```python
from build123d import *

# Parameters (mm, degrees)
SKETCH1_R           = 12.1
BOSS_EXTRUDE1_DEPTH = 31
SKETCH2_R           = 12.65
BOSS_EXTRUDE2_DEPTH = 19
SKETCH3_R           = 3.5
BOSS_EXTRUDE3_DEPTH = 2
SKETCH4_R           = 2
BOSS_EXTRUDE4_DEPTH = 12
SKETCH5_R           = 1.5
CUT_EXTRUDE1_DEPTH  = 6
CUT_EXTRUDE2_START  = -10
CUT_EXTRUDE2_DEPTH  = 10


with BuildPart() as part:
    # Sketch1 → Boss-Extrude1 (new body)
    with BuildSketch(Plane(origin=(0, 0, 0), x_dir=(1, 0, 0), z_dir=(0, 1, 0))):
        with Locations(Location((0, 0, 0), (0, 0, 270))):
            Circle(SKETCH1_R)
    extrude(amount=BOSS_EXTRUDE1_DEPTH)

    # Sketch2 → Boss-Extrude2 (add)
    with BuildSketch(Plane(origin=(0, 31, 0), x_dir=(1, 0, 0), z_dir=(0, 1, 0))):
        with Locations(Location((0, 0, 0), (0, 0, 270))):
            Circle(SKETCH2_R)
    extrude(amount=BOSS_EXTRUDE2_DEPTH)

    # Sketch3 → Boss-Extrude3 (add)
    with BuildSketch(Plane(origin=(0, 50, 0), x_dir=(1, 0, 0), z_dir=(0, 1, 0))):
        with Locations(Location((0, 0, 0), (0, 0, 270))):
            Circle(SKETCH3_R)
    extrude(amount=BOSS_EXTRUDE3_DEPTH)

    # Sketch4 → Boss-Extrude4 (add)
    with BuildSketch(Plane(origin=(0, 52, 0), x_dir=(1, 0, 0), z_dir=(0, 1, 0))):
        with Locations(Location((0, 0, 0), (0, 0, 270))):
            Circle(SKETCH4_R)
    extrude(amount=BOSS_EXTRUDE4_DEPTH)

    # Sketch5 → Cut-Extrude1 (cut)
    with BuildSketch(Plane(origin=(0, 50, 0), x_dir=(1, 0, 0), z_dir=(0, 1, 0))):
        with Locations(Location((8.25, 0, 0), (0, 0, 270))):
            Circle(SKETCH5_R)
        with Locations(Location((-8.25, 0, 0), (0, 0, 270))):
            Circle(SKETCH5_R)
    extrude(amount=-CUT_EXTRUDE1_DEPTH, mode=Mode.SUBTRACT)

    # Sketch6 → Cut-Extrude2 (cut)
    with BuildSketch(Plane(origin=(0, 64, 0), x_dir=(1, 0, 0), z_dir=(0, 1, 0)).offset(CUT_EXTRUDE2_START)):
        with BuildLine():
            Line((-1.428285686, 1.4), (1.428285686, 1.4))
            ThreePointArc((1.428285686, 1.4), (0, 2), (-1.428285686, 1.4))
        make_face()
    extrude(amount=CUT_EXTRUDE2_DEPTH, mode=Mode.SUBTRACT)


solid = part.part
```
Input: part model. Units: mm. Frame: model coordinates. A direction names the side the tool comes from. Give positions to 0.01 mm unless a question says otherwise; leave off trailing zeros. Loops run counter-clockwise (first coordinate to the right, second up) from the corner with the lowest first, then second, coordinate; pieces in that order, holes last. Notation, with made-up numbers: M 16.5,22 L 70.5,22 A25 cw 70.5,44 Z; hole C 4.5,71 d11. An arc over 180 degrees is marked long. Answer as CSV lines item,"result". Start each with the question number.
1. Section B-B on z = -9. Return loops of the section in (x, y).
2. Pull-direction query (X, two-part tool) for faces 5 (the face through (-0.766, 57.916, 1.847)), 6 (the face through (6.786, 47.042, -0.325)), 7 (the face through (0, 64, 0)); classes: released by +X, released by -X, zero draft, split by the parting line, or undercut.
3. Section A-A on x = 0. Return loops of the section in (y, z), plus the area to 3 significant figures.
4. Reachability of faces 1 (the face through (0, 0, 0)), 2 (the face through (-3.417, 50.986, -0.759)), 3 (the face through (0, 59, -1.4)), 4 (the face through (3.635, 15.283, 11.541)) from +Z, -Z, +X, -X, +Y, -Y: full face, straight path, thin tool, end or side. Return the list, or none.
5. Section C-C on y = 5. Return loops of the section in (x, z).
6. Pin query (flat end, axial travel): P1, Ø2, axis at x = -0.5, y = 20, coming from the -Z side; P2, Ø10, axis at y = 34, z = 6.5, coming from the +X side; P3, Ø5, axis at x = -8.25, z = 0, coming from the +Y side. Return the tip coordinate at first contact, or that it passes through.
7. Section D-D on z = 0. Return loops of the section in (x, y).
8. Line query: L1, parallel to X at y = 45.65, z = 0; L2, parallel to Y at x = 6.25, z = -8; L3, parallel to Y at x = 6.5, z = 10.5. Output: solid intervals per line, ascending.
Computed values:
1,outline,"M -8.89,31 L -8.09,31 L -8.09,0 L 8.09,0 L 8.09,31 L 8.89,31 L 8.89,50 L -8.89,50 Z"
2,face 5,"split by the parting line"
2,face 6,"undercut"
2,face 7,"zero draft"
3,outline,"M 0,-12.1 L 31,-12.1 L 31,-12.65 L 50,-12.65 L 50,-3.5 L 52,-3.5 L 52,-2 L 54,-2 L 54,-1.4 L 64,-1.4 L 64,2 L 52,2 L 52,3.5 L 50,3.5 L 50,12.65 L 31,12.65 L 31,12.1 L 0,12.1 Z"
3,area,"1,290 mm²"
4,face 1,"+Z, -Z, +X, -X, -Y"
4,face 2,"+Y"
4,face 3,"-Z, +X, -X, +Y"
4,face 4,"-Y"
5,outline,"C 0,0 d24.2"
6,P1,"stops at z = -12.1"
6,P2,"stops at x = 12.56"
6,P3,"stops at y = 50"
7,outline,"M -12.65,31 L -12.1,31 L -12.1,0 L 12.1,0 L 12.1,31 L 12.65,31 L 12.65,50 L 9.75,50 L 9.75,44 L 6.75,44 L 6.75,50 L 3.5,50 L 3.5,52 L 2,52 L 2,64 L -2,64 L -2,52 L -3.5,52 L -3.5,50 L -6.75,50 L -6.75,44 L -9.75,44 L -9.75,50 L -12.65,50 Z"
8,L1,"x = -12.65 to -9.75, -6.75 to 6.75, 9.75 to 12.65"
8,L2,"y = 0 to 50"
8,L3,"y = 31 to 50"
